```python
from build123d import *

# Parameters (mm, degrees)
SKETCH_1_W          = 47.5
SKETCH_1_H          = 28.5
EXTRUDE_1_DEPTH     = 2.5
SKETCH_2_W          = 45
SKETCH_2_H          = 26
EXTRUDE_2_DEPTH     = 15
SKETCH_3_W          = 36
SKETCH_3_H          = 18
CUT_EXTRUDE_1_DEPTH = 3
CHAMFER_1_SIZE      = 2


with BuildPart() as part:
    # 草图1 → 凸台-拉伸1 (new body)
    with BuildSketch(Plane(origin=(0, 0, 0), x_dir=(1, 0, 0), z_dir=(0, 1, 0))):
        with Locations((23.75, 14.25)):
            Rectangle(SKETCH_1_W, SKETCH_1_H)
    extrude(amount=EXTRUDE_1_DEPTH)

    # 草图2 → 凸台-拉伸2 (add)
    with BuildSketch(Plane(origin=(0, 2.5, 0), x_dir=(1, 0, 0), z_dir=(0, 1, 0))):
        with Locations((23.75, 14.25)):
            Rectangle(SKETCH_2_W, SKETCH_2_H)
    extrude(amount=EXTRUDE_2_DEPTH)

    # 草图3 → 切除-拉伸1 (cut)
    with BuildSketch(Plane.XZ):
        with Locations((23.75, -14.25)):
            Rectangle(SKETCH_3_W, SKETCH_3_H)
    extrude(amount=-CUT_EXTRUDE_1_DEPTH, mode=Mode.SUBTRACT)

    # 倒角1
    chamfer_1_edges = [part.edges().sort_by_distance(p)[0] for p in [
        (41.75, 0, -14.25),
        (23.75, 0, -5.25),
        (5.75, 0, -14.25),
        (23.75, 0, -23.25),
    ]]
    chamfer(chamfer_1_edges, length=CHAMFER_1_SIZE)


solid = part.part
```
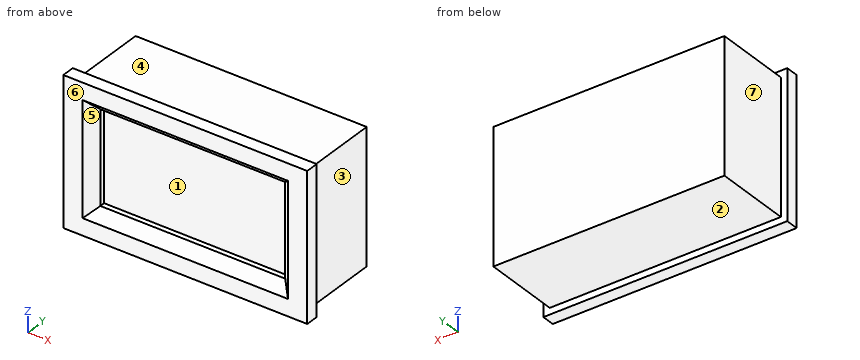
Model file for the job. Use its own axes, mm. Face numbers are marked on the shaded views. A direction names the side the tool comes from. Coordinates: 2 decimals unless noted, no trailing zeros. Loops run counter-clockwise (first coordinate to the right, second up) from the corner with the lowest first, then second, coordinate; pieces in that order, holes last. Notation, with made-up numbers: (-19.5, 87) - (5.5, 87) arc R19 cw to (5.5, 92) - close; hole circle Ø6 at (-18.75, -23). An arc over 180 degrees is marked (long way). Answer as a JSON object with one key per item and string values. Group by question number.
(1) Cut at D-D (y = 14.25). Give the cut face in (x, z), then the cut area to 3 significant figures.
(2) Cut at A-A (x = 4.5). Give the cut face in (y, z).
(3) Cut at C-C (x = 19.5). Give the cut face in (y, z).
(4) Cut at B-B (z = -14). Give the cut face in (x, y), then the cut area to 3 significant figures.
(5) Probe line 1 along X through (y, z) = (2.25, -19.5); line 2 along Y through (x, z) = (30.5, -11.25); line 3 along Z through (x, y) = (41.5, 3.25). List the from-to ranges inside material, lowest first.
(6) Tool access for the marked faces 1, 2, 3 and 4: list every direction of +Z, -Z, +X, -X, +Y, -Y with a clear straight run to the whole face (end or side of a thin tool).
(7) Two-plate mould, pull along X, no slides. Class the marked faces 5, 6 and 7: released by +X, released by -X, zero draft, split by the parting line, or undercut.
(8) Flat gauge pins, fed straight in: pin 1 (10 mm diameter, centred on y = 13.5, z = -13, fed in from -X); pin 2 (2 mm diameter, centred on x = 38, y = 9.5, fed in from +Z); pin 3 (5 mm diameter, centred on x = 42, y = 13, fed in from -Z). Where does each tip first touch, or does it go through?
Geometry says:
{
 "1": {"outline": "(1.25, -27.25) - (46.25, -27.25) - (46.25, -1.25) - (1.25, -1.25) - close", "area": "1,170 mm^2"},
 "2": {"outline": "(0, -28.5) - (2.5, -28.5) - (2.5, -27.25) - (17.5, -27.25) - (17.5, -1.25) - (2.5, -1.25) - (2.5, 0) - (0, 0) - (0, -3.25) - (0.75, -4) - (0.75, -24.5) - (0, -25.25) - close"},
 "3": {"outline": "(0, -28.5) - (2.5, -28.5) - (2.5, -27.25) - (17.5, -27.25) - (17.5, -1.25) - (2.5, -1.25) - (2.5, 0) - (0, 0) - (0, -3.25) - (2, -5.25) - (3, -5.25) - (3, -23.25) - (2, -23.25) - (0, -25.25) - close"},
 "4": {"outline": "(0, 0) - (3.75, 0) - (5.75, 2) - (5.75, 3) - (41.75, 3) - (41.75, 2) - (43.75, 0) - (47.5, 0) - (47.5, 2.5) - (46.25, 2.5) - (46.25, 17.5) - (1.25, 17.5) - (1.25, 2.5) - (0, 2.5) - close", "area": "682 mm^2"},
 "5": {"line 1": "x = 0 to 5.75, 41.75 to 47.5", "line 2": "y = 3 to 17.5", "line 3": "z = -27.25 to -1.25"},
 "6": {"face 1": "-Y", "face 2": "-Z, +X, -X, +Y", "face 3": "+Z, -Z, +X, +Y", "face 4": "+Z, +X, -X, +Y"},
 "7": {"face 5": "undercut", "face 6": "zero draft", "face 7": "released by -X"},
 "8": {"pin 1": "stops at x = 1.25", "pin 2": "stops at z = -1.25", "pin 3": "stops at z = -27.25"}
}
